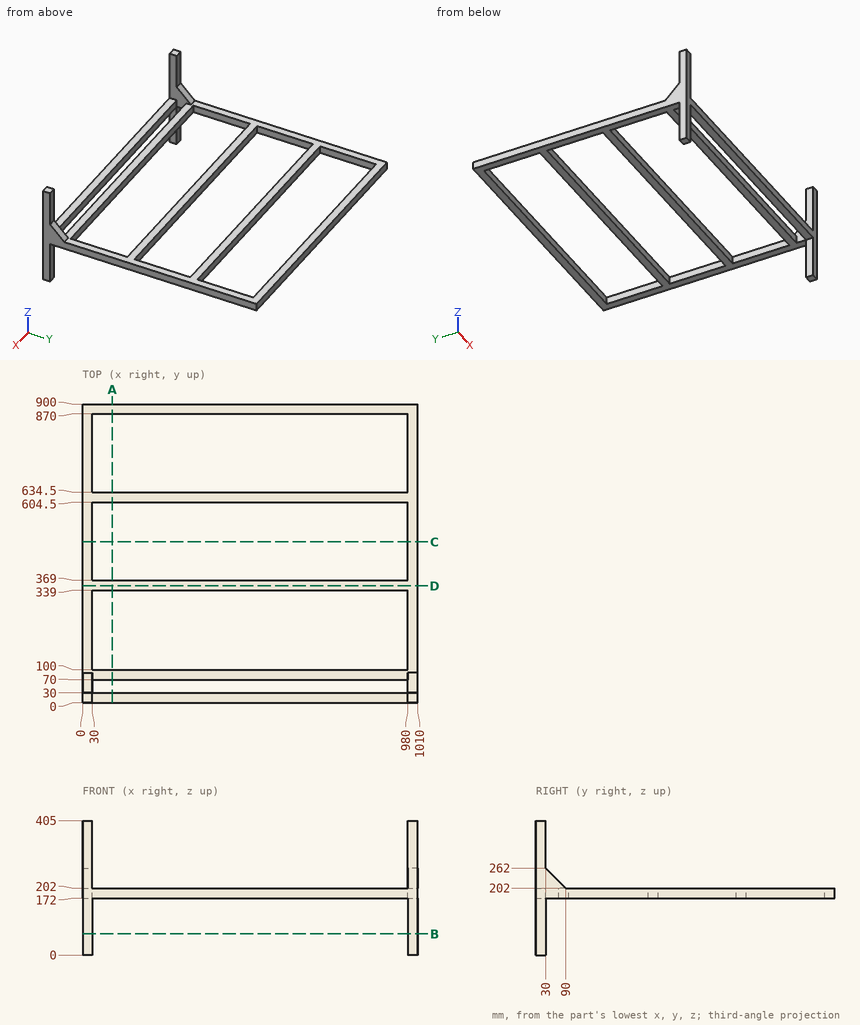
Study the drawing (mm; zero at the part's minimum x, y, z) and answer. Round coordinates to 2 decimals unless told otherwise and drop trailing zeros. Order: outer loops, then holes, each group sorted by start corner. A loop starts at its lowest first (then second) coordinate and runs counter-clockwise, first axis right, second up. Notation, with made-up numbers: M -16,57 L 34,57 A20 cw 34,79 Z; hole C 37,-20.75 d2. An arc over 180 degrees is marked long. One line per item, written item: value.
Q1. Flat-ended cylindrical pins translate along their axes: pin 1 (15 mm diameter, centred on y = 482.5, z = 187, fed in from -X); pin 2 (15 mm diameter, centred on x = 1001, z = 318, fed in from +Y). Find the tip coordinate at first contact, or state that the pin passes through.
Derived:
pin 1: x = 0
pin 2: y = 30
Q2. Find section A-A on x = 90. Write down the section's boundary in (y, z).
Derived:
outline: M 0,172 L 30,172 L 30,202 L 0,202 Z; M 70,172 L 100,172 L 100,202 L 70,202 Z; M 339,172 L 369,172 L 369,202 L 339,202 Z; M 604.5,172 L 634.5,172 L 634.5,202 L 604.5,202 Z; M 870,172 L 900,172 L 900,202 L 870,202 Z
Q3. Straight lines are drawn through the part: line 1 (Y direction, x = 84.5, z = 184.5); line 2 (X direction, y = 66, z = 173); line 3 (Z direction, x = 277, y = 348). For each, find the intervals that lie inside material, in ascending order.
Derived:
line 1: 0 to 30, 70 to 100, 339 to 369, 604.5 to 634.5, 870 to 900
line 2: 0 to 30, 980 to 1010
line 3: 172 to 202
Q4. Find section B-B on z = 64.5. Write down the section's boundary in (x, y), then the cut area to 3 significant figures.
Derived:
outline: M 0,0 L 30,0 L 30,30 L 0,30 Z; M 980,0 L 1010,0 L 1010,30 L 980,30 Z
area: 1,800 mm²
Q5. Find section D-D on y = 352. Write down the section's boundary in (x, z).
Derived:
outline: M 0,172 L 1010,172 L 1010,202 L 0,202 Z
Q6. Find section C-C on y = 485. Write down the section's boundary in (x, z), then the cut area to 3 significant figures.
Derived:
outline: M 0,172 L 30,172 L 30,202 L 0,202 Z; M 980,172 L 1010,172 L 1010,202 L 980,202 Z
area: 1,800 mm²
